Part model, mm, in its own coordinate system. A direction names the side the tool comes from. Coordinates: 2 decimals unless noted, no trailing zeros. Loops run counter-clockwise (first coordinate to the right, second up) from the corner with the lowest first, then second, coordinate; pieces in that order, holes last. Notation, with made-up numbers: (40, 45.25) -> (56, 45.25) arc R15 cw to (56, 59.25) -> close; hole circle Ø2 at (-2.5, 12.5). An arc over 180 degrees is marked (long way). Use one line per item in the form item = value. Start each with the question number.
(1) Band-saw the part on C-C on y = -0.5. Give the cut face in (x, z).
(2) Mould opens along Y. For faces 1 (the flat face through (0, 0, 0)), 2 (the cylindrical face through (-3.33, -2.93, 1.48)), 3 (the cylindrical face through (-1.5, -4.2, 1.5)) say: +Y half, -Y half, draft (parallel to the pull), parting line (faces both ways), or undercut.
(3) Band-saw the part on B-B on x = 0.25. Give the cut face in (y, z).
(4) 3-axis set-ups, long thin cutter, end or side, ignore diameter. For faces 4 (the flat face through (-3, 0, 1)), 5 (the cylindrical face through (4.004, 1.869, 1.479)), 6 (the flat face through (2.978, -1.294, 1.479)): which of +Z, -Z, +X, -X, +Y, -Y reach the whole face in a straight line?
(5) Pin check, flat tips, straight feed: P1, Ø1.1, axis at x = -3, z = 1.5, coming from the -Y side; P2, Ø0.8, axis at x = 3.5, z = 1, coming from the +Y side; P3, Ø2, axis at x = -3.5, y = -1, coming from the -Z side; P4, Ø1.5, axis at x = 1.5, z = 2, coming from the -Y side. Stop position of each tip, or through.
(6) Drill centre lines: L1, parallel to X at y = -4, z = 2.6; L2, parallel to Y at x = 0.5, z = 2.65; L3, parallel to Y at x = 1.75, z = 1.65. Where is each one in solid material? Low to high. Write a range as [from, to].
(7) Band-saw the part on A-A on y = 2.25. Give the cut face in (x, z), then the cut area to 3 significant figures.
```python
from build123d import *

# Parameters (mm, degrees)
BOSS_EXTRU_1_DEPTH           = 3
R_P_TITION_CIRCULAIRE2_COUNT = 8
ESQUISSE5_R                  = 2.75
BOSS_EXTRU_2_DEPTH           = 3


with BuildPart() as part:
    # Esquisse4 → Boss.-Extru.1 (new body)
    with BuildSketch(Plane.XY):
        with BuildLine():
            Line((0, 3.758770483), (0, 2.75))
            ThreePointArc((0, 2.75), (0.559711277, 2.692438168), (1.095991276, 2.52216239))
            Line((1.095991276, 2.52216239), (1.498028967, 3.447356198))
            ThreePointArc((1.498028967, 3.447356198), (1.508290586, 4.162952408), (1.26714265, 4.836770566))
            ThreePointArc((1.26714265, 4.836770566), (1.017656867, 4.895342123), (0.765497749, 4.941053855))
            ThreePointArc((0.765497749, 4.941053855), (0.275783903, 4.419169208), (0, 3.758770483))
        make_face()
    extrude(amount=BOSS_EXTRU_1_DEPTH)


with BuildPart() as r_p_tition_circulaire2_1:
    # R_p_tition circulaire2: pattern copy
    add(part.part.rotate(Axis((0, 0, 0), (0, 0, 1)), 1 * 360 / R_P_TITION_CIRCULAIRE2_COUNT))


with BuildPart() as r_p_tition_circulaire2_2:
    # R_p_tition circulaire2: pattern copy
    add(part.part.rotate(Axis((0, 0, 0), (0, 0, 1)), 2 * 360 / R_P_TITION_CIRCULAIRE2_COUNT))


with BuildPart() as r_p_tition_circulaire2_3:
    # R_p_tition circulaire2: pattern copy
    add(part.part.rotate(Axis((0, 0, 0), (0, 0, 1)), 3 * 360 / R_P_TITION_CIRCULAIRE2_COUNT))


with BuildPart() as r_p_tition_circulaire2_4:
    # R_p_tition circulaire2: pattern copy
    add(part.part.rotate(Axis((0, 0, 0), (0, 0, 1)), 4 * 360 / R_P_TITION_CIRCULAIRE2_COUNT))


with BuildPart() as r_p_tition_circulaire2_5:
    # R_p_tition circulaire2: pattern copy
    add(part.part.rotate(Axis((0, 0, 0), (0, 0, 1)), 5 * 360 / R_P_TITION_CIRCULAIRE2_COUNT))


with BuildPart() as r_p_tition_circulaire2_6:
    # R_p_tition circulaire2: pattern copy
    add(part.part.rotate(Axis((0, 0, 0), (0, 0, 1)), 6 * 360 / R_P_TITION_CIRCULAIRE2_COUNT))


with BuildPart() as r_p_tition_circulaire2_7:
    # R_p_tition circulaire2: pattern copy
    add(part.part.rotate(Axis((0, 0, 0), (0, 0, 1)), 7 * 360 / R_P_TITION_CIRCULAIRE2_COUNT))


with BuildPart() as part_1:
    add(part.part)

    add(r_p_tition_circulaire2_1.part)  # Boss.-Extru.2 merges R_p_tition circulaire2_1

    add(r_p_tition_circulaire2_2.part)  # Boss.-Extru.2 merges R_p_tition circulaire2_2

    add(r_p_tition_circulaire2_3.part)  # Boss.-Extru.2 merges R_p_tition circulaire2_3

    add(r_p_tition_circulaire2_4.part)  # Boss.-Extru.2 merges R_p_tition circulaire2_4

    add(r_p_tition_circulaire2_5.part)  # Boss.-Extru.2 merges R_p_tition circulaire2_5

    add(r_p_tition_circulaire2_6.part)  # Boss.-Extru.2 merges R_p_tition circulaire2_6

    add(r_p_tition_circulaire2_7.part)  # Boss.-Extru.2 merges R_p_tition circulaire2_7
    # Esquisse5 → Boss.-Extru.2 (add)
    with BuildSketch(Plane.XY):
        Circle(ESQUISSE5_R)
    extrude(amount=BOSS_EXTRU_2_DEPTH)


solid = part_1.part
```
A:
q1.outline = (-2.7, 0) -> (4.71, 0) -> (4.71, 3) -> (-2.7, 3) -> close
q2.face_1 = draft
q2.face_2 = -Y half
q2.face_3 = undercut
q3.outline = (-2.74, 0) -> (4.38, 0) -> (4.38, 3) -> (-2.74, 3) -> close
q4.face_4 = +Z, -Z, -X
q4.face_5 = +Z, -Z, +X
q4.face_6 = +Z, -Z
q5.P1 = -2.97
q5.P2 = 2.97
q5.P3 = 0
q5.P4 = -4.22
q6.L1 = [-1.53, -0.07], [1.86, 2.96]
q6.L2 = [-2.7, 4.71]
q6.L3 = [-3.91, 2.12]
q7.outline = (-2.25, 0) -> (1.58, 0) -> (1.58, 3) -> (-2.25, 3) -> close; (2.25, 0) -> (4.22, 0) -> (4.22, 3) -> (2.25, 3) -> close
q7.area = 17.4 mm²
